Could you check a few things on this drawing? It's one solid part, dimensions in mm from its lowest x, y, z. Give positions to 0.01 mm unless a question says otherwise; leave off trailing zeros. Order: outer loops, then holes, each group sorted by start corner. A loop starts at its lowest first (then second) coordinate and runs counter-clockwise, first axis right, second up.
Item 1: I want a section at B-B, the plane z = 98.99. Write out the boundary of the cut face in (x, y), then the cut area to 3 significant figures.
Item 2: I want a section at D-D, the plane x = 164.5. Write out the boundary of the cut face in (y, z).
Item 3: I want a section at A-A, the plane y = 6.75. Write out the boundary of the cut face in (x, z), then the cut area to 3 significant figures.
Item 4: I want a section at C-C, the plane x = 39. Write out the boundary of the cut face in (y, z), then the cut area to 3 significant figures.
Item 5: I'm going to push flat-ended pins straight in: pin 1 Ø11 at (x, z) = (95, 98.99) entering from +Y; pin 2 Ø5 at (y, z) = (2, 205.5) entering from +X. Where does each tip first touch, or does it pass through?
Item 6: If I drill on line 1 along Z through (x, y) = (164.5, 2.5); line 2 along Z through (x, y) = (38.5, 7.5); line 3 along X through (y, z) = (5.5, 162.99), over which ranges is the centre line in solid material (lowest first)?
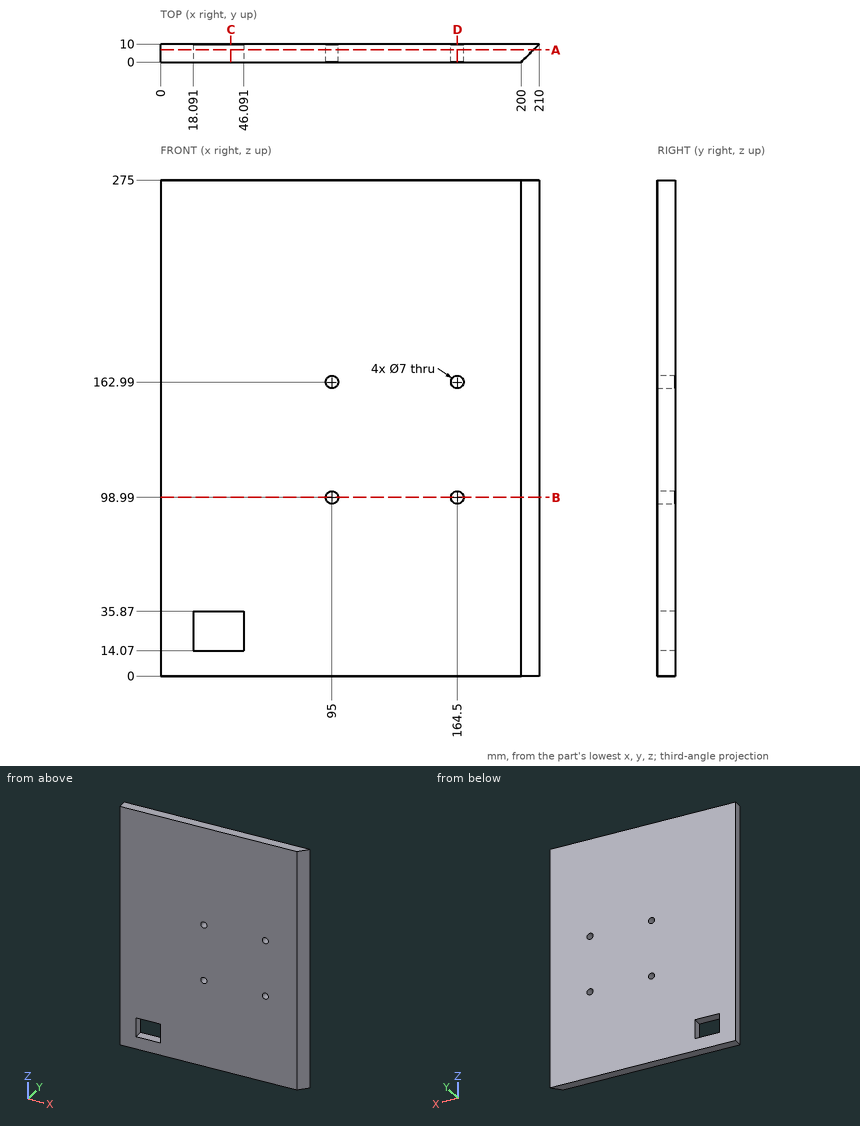
Results list:
1. outline: (0, 0) - (91.5, 0) - (91.5, 10) - (0, 10) - close; (98.5, 0) - (161, 0) - (161, 10) - (98.5, 10) - close; (168, 0) - (200, 0) - (210, 10) - (168, 10) - close
1. area: 1,910 mm2
2. outline: (0, 0) - (10, 0) - (10, 95.49) - (0, 95.49) - close; (0, 102.49) - (10, 102.49) - (10, 159.49) - (0, 159.49) - close; (0, 166.49) - (10, 166.49) - (10, 275) - (0, 275) - close
3. outline: (0, 0) - (206.75, 0) - (206.75, 275) - (0, 275) - close; hole (18.09, 14.07) - (46.09, 14.07) - (46.09, 35.87) - (18.09, 35.87) - close; hole circle Ø7 at (95, 98.99); hole circle Ø7 at (95, 162.99); hole circle Ø7 at (164.5, 98.99); hole circle Ø7 at (164.5, 162.99)
3. area: 56,100 mm2
4. outline: (0, 0) - (10, 0) - (10, 14.07) - (0, 14.07) - close; (0, 35.87) - (10, 35.87) - (10, 275) - (0, 275) - close
4. area: 2,530 mm2
5. pin 1: stops at y = 10
5. pin 2: stops at x = 204.5
6. line 1: z = 0 to 95.49, 102.49 to 159.49, 166.49 to 275
6. line 2: z = 0 to 14.07, 35.87 to 275
6. line 3: x = 0 to 91.5, 98.5 to 161, 168 to 205.5
